For this review, take the finished solid that the model builds, in its own axes (mm). Face numbers are marked on the shaded views. A direction names the side the tool comes from. Coordinates: 2 decimals unless noted, no trailing zeros. Order: outer loops, then holes, each group sorted by start corner. A loop starts at its lowest first (then second) coordinate and runs counter-clockwise, first axis right, second up. Notation, with made-up numbers: M 60,38.5 L 86,38.5 A19 cw 86,51.5 Z; hole C 48,5 d10. An arc over 180 degrees is marked long. Use CSV: the item, a comma, the result in double quotes.
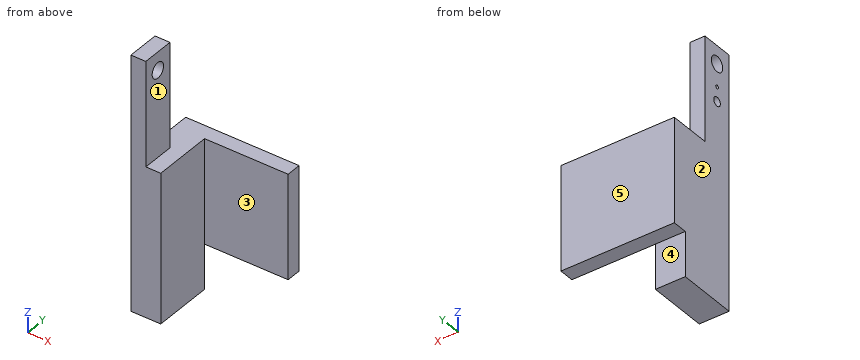
```python
from build123d import *

# Parameters (mm, degrees)
SKETCH_1_W          = 38
SKETCH_1_H          = 35
EXTRUDE_1_DEPTH     = 5
SKETCH_1_14_W       = 10
SKETCH_1_14_H       = 50
EXTRUDE_2_DEPTH     = 20
EXTRUDE_START       = -5
SKETCH_2_W          = 35
SKETCH_2_H          = 11
SKETCH_2_R          = 2.6
EXTRUDE_3_DEPTH     = 5
CUT_EXTRUDE_START   = -10
SKETCH_2_3_R        = 0.6
SKETCH_2_3_R_2      = 1.5
CUT_EXTRUDE_1_DEPTH = 3


with BuildPart() as part:
    # 草图1 → 凸台-拉伸1 (new body)
    with BuildSketch(Plane(origin=(0, 0, 0), x_dir=(1, 0, 0), z_dir=(0, 1, 0))):
        with Locations((19, -17.5)):
            Rectangle(SKETCH_1_W, SKETCH_1_H)
    extrude(amount=EXTRUDE_1_DEPTH)

    # 草图1<14> → 凸台-拉伸2 (add)
    with BuildSketch(Plane(origin=(0, 0, 0), x_dir=(1, 0, 0), z_dir=(0, 1, 0))):
        with Locations((5, -10)):
            Rectangle(SKETCH_1_14_W, SKETCH_1_14_H)
    extrude(amount=-EXTRUDE_2_DEPTH)

    # 草图2 → 凸台-拉伸3 (add)
    with BuildSketch(Plane(origin=(10, 0, 0), x_dir=(0, 0, -1), z_dir=(1, 0, 0)).offset(EXTRUDE_START)):
        with Locations((-52.5, -14.5)):
            Rectangle(SKETCH_2_W, SKETCH_2_H)
        with Locations((-63.9, -14.5)):
            Circle(SKETCH_2_R, mode=Mode.SUBTRACT)
    extrude(amount=-EXTRUDE_3_DEPTH)

    # 草图2<3> → 切除-拉伸1 (cut)
    with BuildSketch(Plane(origin=(10, 0, 0), x_dir=(0, 0, -1), z_dir=(1, 0, 0)).offset(CUT_EXTRUDE_START)):
        with Locations((-56.3, -14.5)):
            Circle(SKETCH_2_3_R)
        with Locations((-51.4, -14.5)):
            Circle(SKETCH_2_3_R_2)
    extrude(amount=CUT_EXTRUDE_1_DEPTH, mode=Mode.SUBTRACT)


solid = part.part
```
Item 1: Clearance check with flat-ended pins moving along their axes: pin 1 Ø14 at (x, z) = (30.5, 25.5) entering from -Y; pin 2 Ø1 at (x, y) = (31.5, 1.5) entering from -Z; pin 3 Ø5 at (x, z) = (5, -9) entering from +Y. State where each tip first meets the part, or that it passes through.
Solutions:
pin 1,"y = 0"
pin 2,"z = 0"
pin 3,"y = 0"
Item 2: Add section A-A on x = 4. State the section outline as (y, z) points.
Solutions:
outline,"M -20,-15 L 0,-15 L 0,0 L 5,0 L 5,35 L -9,35 L -9,70 L -20,70 Z; hole C -14.5,63.9 d5.2"
Item 3: Add section B-B on z = 63.9. State the section outline as (x, y) points, and give its area (3 significant figures).
Solutions:
outline,"M 0,-20 L 5,-20 L 5,-17.1 L 0,-17.1 Z; M 0,-11.9 L 5,-11.9 L 5,-9 L 0,-9 Z"
area,"29.0 mm^2"
Item 4: To check wall thickness, follow line 1 along Y through (x, z) = (1.75, 51.4); line 2 along Y through (x, z) = (3.75, 63.9); line 3 along X through (y, z) = (-12.25, 40). State the ranges of each line that lie inside material, in increasing order. Write a range as [from, to].
Solutions:
line 1,"[-20, -16], [-13, -9]"
line 2,"[-20, -17.1], [-11.9, -9]"
line 3,"[0, 5]"
Item 5: Add section D-D on x = 19.5. State the section outline as (y, z) points.
Solutions:
outline,"M 0,0 L 5,0 L 5,35 L 0,35 Z"
Item 6: Add section C-C on z = 51.4. State the section outline as (x, y) points, and give its area (3 significant figures).
Solutions:
outline,"M 0,-20 L 5,-20 L 5,-9 L 0,-9 L 0,-13 L 3,-13 L 3,-16 L 0,-16 Z"
area,"46.0 mm^2"
Item 7: For the marked faces 1, 2, 3, 4 and 5, list the 3-axis set-ups (+Z, -Z, +X, -X, +Y, -Y) from which the entire face can be reached by the end or side of a thin tool; tool diameter is ignored.
Solutions:
face 1,"+Z, +X, +Y, -Y"
face 2,"+Z, -Z, -X, +Y, -Y"
face 3,"+Z, -Z, +X, -Y"
face 4,"-Z, +X, -X, +Y"
face 5,"+Z, -Z, +X, -X, +Y"
